Job drawing, mm, ordinate dimensions from the low corner. One solid piece. A direction names the side the tool comes from. Give positions to 0.01 mm unless a question says otherwise; leave off trailing zeros. Order: outer loops, then holes, each group sorted by start corner. A loop starts at its lowest first (then second) coordinate and runs counter-clockwise, first axis right, second up. Notation, with made-up numbers: (-15, 67.5) - (31, 67.5) arc R6 ccw to (31, 71.5) - close; hole circle Ø6 at (-13, -19). An arc over 180 degrees is marked (long way). Write each question's results on one line, items separated by ' | '. Start each with the question number.
1) Two-plate mould, pull along X, no slides. Class the marked faces 1, 2, 3 and 4: +X half, -X half, draft (parallel to the pull), parting line (faces both ways), or undercut.
2) Cut at D-D on z = 73.5. List the corners of the cut face in (x, y).
3) Tool access for the marked faces 5, 6 and 7: list every direction of +Z, -Z, +X, -X, +Y, -Y with a clear straight run to the whole face (end or side of a thin tool).
4) Drop flat-ended pins along their axis: pin 1 Ø12 at (y, z) = (144.5, 71) entering from +X; pin 2 Ø10 at (x, z) = (50, 70.5) entering from -Y; pin 3 Ø24 at (x, y) = (52, 100) entering from +Z. Give the stop position or say it passes through.
5) Cut at C-C on x = 110. List the corners of the cut face in (y, z).
6) Drill centre lines: line 1 along Z through (x, y) = (110, 191); line 2 along X through (y, z) = (130, 80); line 3 along X through (y, z) = (130, 25.5). Where is each one in solid material? Low to high. Write a range as from..to.
7) Cut at B-B on y = 130. List the corners of the cut face in (x, z).
8) Cut at A-A on z = 90. List the corners of the cut face in (x, y).
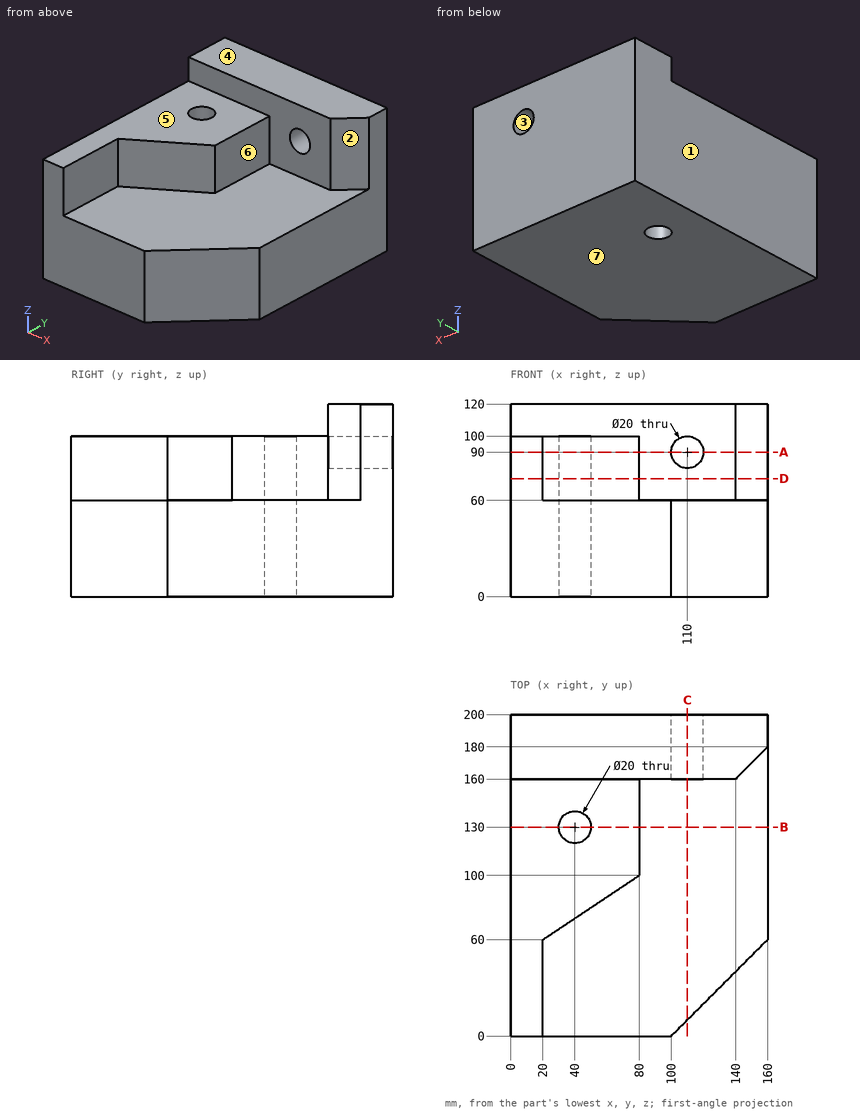
Results:
1) face 1: -X half | face 2: +X half | face 3: undercut | face 4: draft
2) outline: (0, 0) - (20, 0) - (20, 60) - (80, 100) - (80, 160) - (140, 160) - (160, 180) - (160, 200) - (0, 200) - close; hole circle Ø20 at (40, 130)
3) face 5: +Z, +X, -X, -Y | face 6: +Z, +X, -Y | face 7: -Z, +X, -X, +Y, -Y
4) pin 1: x = 80 | pin 2: y = 76.67 | pin 3: z = 100
5) outline: (10, 0) - (200, 0) - (200, 80) - (160, 80) - (160, 60) - (10, 60) - close; (160, 100) - (200, 100) - (200, 120) - (160, 120) - close
6) line 1: 0..80, 100..120 | line 2: 0..30, 50..80 | line 3: 0..30, 50..160
7) outline: (0, 0) - (30, 0) - (30, 100) - (0, 100) - close; (50, 0) - (160, 0) - (160, 60) - (80, 60) - (80, 100) - (50, 100) - close
8) outline: (0, 0) - (20, 0) - (20, 60) - (80, 100) - (80, 160) - (100, 160) - (100, 200) - (0, 200) - close; (120, 160) - (140, 160) - (160, 180) - (160, 200) - (120, 200) - close; hole circle Ø20 at (40, 130)
